```python
from build123d import *

# Parameters (mm, degrees)
F1_DEPTH       = 90
F3_D           = 4.4
F3_CBORE_D     = 8.25
F3_CBORE_DEPTH = 4
F4_R           = 5
F5_T1_DEPTH    = 88
F5_T3_DEPTH    = 26.5
F5_T5_DEPTH    = 48
F5_S9_W        = 1
F5_S9_H        = 1
F5_T10_DEPTH   = 1
F5_S15_W       = 1
F5_S15_H       = 1
F5_T16_DEPTH   = 1
F5_S21_W       = 1
F5_S21_H       = 1
F5_T22_DEPTH   = 1
F5_S27_W       = 1
F5_S27_H       = 1
F5_T28_DEPTH   = 1


# Not quite as in the source:
# - a fillet or chamfer that OpenCascade refuses, or shapes differently, is made with other operations: its cross-section is extruded or revolved along the edge and cut away or added


with BuildPart() as f1:
    # F0 (on Front) → F1 (new body)
    with BuildSketch(Plane.XZ):
        with BuildLine():
            Line((25, 0), (25, 25))
            Line((25, 25), (-25, 25))
            Line((-25, 25), (-25, 0))
            Line((-25, 0), (-16, 0))
            ThreePointArc((-16, 0), (0, 16), (16, 0))
            Line((16, 0), (25, 0))
        make_face()
    extrude(amount=F1_DEPTH)

    # F3 (through all)
    with Locations(Plane.XY.offset(25)):
        with Locations((-20, -85), (-20, -5), (20, -5), (20, -85)):
            CounterBoreHole(F3_D / 2, F3_CBORE_D / 2, F3_CBORE_DEPTH)

    # F4
    f4_edges = [f1.edges().sort_by_distance(p)[0] for p in [
        (0, -90, 16),
    ]]
    fillet(f4_edges, radius=F4_R)

    # F5: fillet of radius 1 on 8 edges, made by hand

    # F5_s2 → F5_t1 (cut)
    with BuildSketch(Plane.XZ.offset(1)):
        with BuildLine():
            ThreePointArc((25, 24), (24.7071067812, 24.7071067812), (24, 25))
            Line((24, 25), (25, 25))
            Line((25, 25), (25, 24))
        make_face()
        with BuildLine():
            ThreePointArc((-24, 25), (-24.7071067812, 24.7071067812), (-25, 24))
            Line((-25, 24), (-25, 25))
            Line((-25, 25), (-24, 25))
        make_face()
    extrude(amount=F5_T1_DEPTH, mode=Mode.SUBTRACT)

    # F5_s4 → F5_t3 (cut)
    with BuildSketch(Plane.XY.offset(-2.5)):
        with BuildLine():
            ThreePointArc((24, -90), (24.7071067812, -89.7071067812), (25, -89))
            Line((25, -89), (25, -90))
            Line((25, -90), (24, -90))
        make_face()
        with BuildLine():
            ThreePointArc((24, 0), (24.7071067812, -0.2928932188), (25, -1))
            Line((25, -1), (25, 0))
            Line((25, 0), (24, 0))
        make_face()
        with BuildLine():
            ThreePointArc((-24, 0), (-24.7071067812, -0.2928932188), (-25, -1))
            Line((-25, -1), (-25, 0))
            Line((-25, 0), (-24, 0))
        make_face()
        with BuildLine():
            ThreePointArc((-24, -90), (-24.7071067812, -89.7071067812), (-25, -89))
            Line((-25, -89), (-25, -90))
            Line((-25, -90), (-24, -90))
        make_face()
    extrude(amount=F5_T3_DEPTH, mode=Mode.SUBTRACT)

    # F5_s6 → F5_t5 (cut)
    with BuildSketch(Plane.YZ.offset(-24)):
        with BuildLine():
            ThreePointArc((0, 24), (-0.2928932188, 24.7071067812), (-1, 25))
            Line((-1, 25), (0, 25))
            Line((0, 25), (0, 24))
        make_face()
        with BuildLine():
            ThreePointArc((-90, 24), (-89.7071067812, 24.7071067812), (-89, 25))
            Line((-89, 25), (-90, 25))
            Line((-90, 25), (-90, 24))
        make_face()
    extrude(amount=F5_T5_DEPTH, mode=Mode.SUBTRACT)


with BuildPart() as f5_tool8:
    # F5_s9 → F5_t10 (new body)
    with BuildSketch(Plane.XY.offset(24)):
        with Locations((24.5, -0.5)):
            Rectangle(F5_S9_W, F5_S9_H)
    extrude(amount=F5_T10_DEPTH)

    # F5_s11 → F5_t12 (revolve, cut)
    with BuildSketch(Plane(origin=(24, -1, 24), x_dir=(-0.7071067812, -0.7071067812, 0), z_dir=(-0.7071067812, 0.7071067812, 0))):
        with BuildLine():
            ThreePointArc((0, -1), (1, 0), (0, 1))
            Line((0, 1), (0, -1))
        make_face()
    revolve(axis=Axis((24, -1, 24), (0, 0, 1)), mode=Mode.SUBTRACT)


with BuildPart() as f1_1:
    add(f1.part)

    # F5_t7: cut F5_tool8
    add(f5_tool8.part, mode=Mode.SUBTRACT)


with BuildPart() as f5_tool14:
    # F5_s15 → F5_t16 (new body)
    with BuildSketch(Plane.XY.offset(24)):
        with Locations((24.5, -89.5)):
            Rectangle(F5_S15_W, F5_S15_H)
    extrude(amount=F5_T16_DEPTH)

    # F5_s17 → F5_t18 (revolve, cut)
    with BuildSketch(Plane(origin=(24, -89, 24), x_dir=(-0.7071067812, 0.7071067812, 0), z_dir=(0.7071067812, 0.7071067812, 0))):
        with BuildLine():
            ThreePointArc((0, -1), (1, 0), (0, 1))
            Line((0, 1), (0, -1))
        make_face()
    revolve(axis=Axis((24, -89, 24), (0, 0, 1)), mode=Mode.SUBTRACT)


with BuildPart() as f1_2:
    add(f1_1.part)

    # F5_t13: cut F5_tool14
    add(f5_tool14.part, mode=Mode.SUBTRACT)


with BuildPart() as f5_tool20:
    # F5_s21 → F5_t22 (new body)
    with BuildSketch(Plane.XY.offset(24)):
        with Locations((-24.5, -0.5)):
            Rectangle(F5_S21_W, F5_S21_H)
    extrude(amount=F5_T22_DEPTH)

    # F5_s23 → F5_t24 (revolve, cut)
    with BuildSketch(Plane(origin=(-24, -1, 24), x_dir=(0.7071067812, -0.7071067812, 0), z_dir=(-0.7071067812, -0.7071067812, 0))):
        with BuildLine():
            ThreePointArc((0, -1), (1, 0), (0, 1))
            Line((0, 1), (0, -1))
        make_face()
    revolve(axis=Axis((-24, -1, 24), (0, 0, 1)), mode=Mode.SUBTRACT)


with BuildPart() as f1_3:
    add(f1_2.part)

    # F5_t19: cut F5_tool20
    add(f5_tool20.part, mode=Mode.SUBTRACT)


with BuildPart() as f5_tool26:
    # F5_s27 → F5_t28 (new body)
    with BuildSketch(Plane.XY.offset(24)):
        with Locations((-24.5, -89.5)):
            Rectangle(F5_S27_W, F5_S27_H)
    extrude(amount=F5_T28_DEPTH)

    # F5_s29 → F5_t30 (revolve, cut)
    with BuildSketch(Plane(origin=(-24, -89, 24), x_dir=(0.7071067812, 0.7071067812, 0), z_dir=(0.7071067812, -0.7071067812, 0))):
        with BuildLine():
            ThreePointArc((0, -1), (1, 0), (0, 1))
            Line((0, 1), (0, -1))
        make_face()
    revolve(axis=Axis((-24, -89, 24), (0, 0, 1)), mode=Mode.SUBTRACT)


with BuildPart() as f1_4:
    add(f1_3.part)

    # F5_t25: cut F5_tool26
    add(f5_tool26.part, mode=Mode.SUBTRACT)


solid = f1_4.part
```
The listing builds one solid part. Answer for the finished solid, in the listing's coordinates (mm). A direction names the side the tool comes from. Coordinates: 2 decimals unless noted, no trailing zeros. Loops run counter-clockwise (first coordinate to the right, second up) from the corner with the lowest first, then second, coordinate; pieces in that order, holes last. Notation, with made-up numbers: (60.5, 65.25) - (69.5, 65.25) arc R15 ccw to (69.5, 84.25) - close; hole circle Ø9 at (-26, -38). An arc over 180 degrees is marked (long way). Write item = value, one per line.
1) Each of these flat-tipped pins is pushed along its axis until it touches: P1, Ø7.5, axis at x = 20, y = -85, coming from the +Z side; P2, Ø10.5, axis at x = 20, y = -5, coming from the +Z side; P3, Ø6, axis at x = -1.5, y = -41.5, coming from the -Z side; P4, Ø8, axis at x = -10.5, y = -68.5, coming from the -Z side. Where does it stop, or does it pass through?
Responses:
P1 = 21
P2 = 25
P3 = 15.35
P4 = 6.76
2) Determine the mould class of faces 3 (the face through (23.2, -1.8, 25)), 4 (the face through (-21, -81, 23)), 5 (the face through (-25, -44, 12)) for opening direction X: pulls with the +X half, pulls with the -X half, needs draft (parallel to the pull), parting line crosses it, or undercut.
Responses:
face_3 = needs draft
face_4 = undercut
face_5 = pulls with the -X half
3) Section B-B (x = 0) is taken. Determine the outline of the cut face in (y, z), plus the area to 3 significant figures.
Responses:
outline = (-90, 21) arc R5 ccw to (-85, 16) - (0, 16) - (0, 24) arc R1 ccw to (-1, 25) - (-89, 25) arc R1 ccw to (-90, 24) - close
area = 804 mm^2
4) Section C-C (y = -20) is taken. Determine the outline of the cut face in (x, z).
Responses:
outline = (-25, 0) - (-16, 0) arc R16 cw to (16, 0) - (25, 0) - (25, 24) arc R1 ccw to (24, 25) - (-24, 25) arc R1 ccw to (-25, 24) - close
5) Find the intervals of material crossed by line 1 along Y through (x, z) = (20, 23.75) (3 decimals); line 2 along X through (y, z) = (-85, 23.75) (3 decimals); line 3 along Y through (x, z) = (20.5, 9), in increasing order.
Responses:
line_1 = -90 to -89.125, -80.875 to -9.125, -0.875 to 0
line_2 = -25 to -24.125, -15.875 to 15.875, 24.125 to 25
line_3 = -90 to -87.14, -82.86 to -7.14, -2.86 to 0
6) Which of the six approach directions +Z, -Z, +X, -X, +Y, -Y give full straight-line access (tool end or side, diameter ignored) to faces 1 (the face through (0, -42, 16)), 2 (the face through (-23.273, -7.51, 23.028))?
Responses:
face_1 = -Z, +Y, -Y
face_2 = +Z
7) Section A-A (z = 22.25) is taken. Determine the outline of the cut face in (x, y) (3 decimals), plus the area to 3 significant figures.
Responses:
outline = (-25, -89) arc R1 ccw to (-24, -90) - (24, -90) arc R1 ccw to (25, -89) - (25, -1) arc R1 ccw to (24, 0) - (-24, 0) arc R1 ccw to (-25, -1) - close; hole circle Ø8.25 at (-20, -85); hole circle Ø8.25 at (-20, -5); hole circle Ø8.25 at (20, -85); hole circle Ø8.25 at (20, -5)
area = 4,290 mm^2
8) Section D-D (y = -5) is taken. Determine the outline of the cut face in (x, z) (3 decimals).
Responses:
outline = (-25, 0) - (-22.2, 0) - (-22.2, 21) - (-24.125, 21) - (-24.125, 24.992) arc R1 ccw to (-25, 24) - close; (-17.8, 0) - (-16, 0) arc R16 cw to (16, 0) - (17.8, 0) - (17.8, 21) - (15.875, 21) - (15.875, 25) - (-15.875, 25) - (-15.875, 21) - (-17.8, 21) - close; (22.2, 0) - (25, 0) - (25, 24) arc R1 ccw to (24.125, 24.992) - (24.125, 21) - (22.2, 21) - close
